from build123d import *

# Parameters (mm, degrees)
BOSS_EXTRUDE1_DEPTH      = 5
CUT_EXTRUDE1_DEPTH       = 1
BOSS_EXTRUDE2_DEPTH      = 0.0254
BOSS_EXTRUDE2_DEPTH_BACK = 1
SKETCH3_W                = 0.777152918
SKETCH3_H                = 1.679205413


with BuildPart() as part:
    # Sketch1 → Boss-Extrude1 (new body)
    with BuildSketch(Plane(origin=(0, 0, 0), x_dir=(1, 0, 0), z_dir=(0, 1, 0))):
        Polygon((-3, 2), (-2, 3), (2, 3), (3, 2), (3, -2), (2, -3), (-2, -3), (-3, -2), align=None)
    extrude(amount=BOSS_EXTRUDE1_DEPTH)

    # Sketch2 → Cut-Extrude1 (cut)
    with BuildSketch(Plane(origin=(0, 5, 0), x_dir=(1, 0, 0), z_dir=(0, 1, 0))):
        Polygon((3, -2), (3, 2), (2, 3), (-2, 3), (-3, 2), (-3, -2), (-2, -3), (2, -3), align=None)
        Polygon((2.492, -1.78957951), (2.492, 1.78957951), (1.78957951, 2.492), (-1.78957951, 2.492), (-2.492, 1.78957951), (-2.492, -1.78957951), (-1.78957951, -2.492), (1.78957951, -2.492), align=None, mode=Mode.SUBTRACT)
    extrude(amount=-CUT_EXTRUDE1_DEPTH, mode=Mode.SUBTRACT)

    # Sketch3 → Boss-Extrude2 (add, two sides: drawn at the far end of the back side and taken through both)
    with BuildSketch(Plane.XZ.offset(-BOSS_EXTRUDE2_DEPTH_BACK)):
        with Locations((0, 2.210397294)):
            Rectangle(SKETCH3_W, SKETCH3_H)
        with Locations((0, -2.210397294)):
            Rectangle(SKETCH3_W, SKETCH3_H)
    extrude(amount=BOSS_EXTRUDE2_DEPTH + BOSS_EXTRUDE2_DEPTH_BACK)


solid = part.part
The model under review builds one solid part; all positions refer to its coordinate system, in mm. A direction names the side the tool comes from. Give positions to 0.01 mm unless a question says otherwise; leave off trailing zeros. Order: outer loops, then holes, each group sorted by start corner. A loop starts at its lowest first (then second) coordinate and runs counter-clockwise, first axis right, second up. Notation, with made-up numbers: M 24,54.5 L 60,54.5 A33 cw 60,84.5 Z; hole C 61.5,-6.75 d10. An arc over 180 degrees is marked long. Answer in a Markdown table with one row per item. Add a question column.
1. Machinability: for faces 1 (the flat face through (2.492, 4.5, 0)), 2 (the flat face through (-2.492, 4.5, 0)), 3 (the flat face through (0, 4.5, 2.492)), 4 (the flat face through (0, 4.5, -2.492)), 5 (the flat face through (0, 4, -2.7)), which of the approach directions +Z, -Z, +X, -X, +Y, -Y give a long, thin tool a straight path to every point of the face, cutting with its end or side? Answer none if there is none.
2. Add section C-C on y = 4.45. State the section outline as (x, z) points, plus the area to 3 significant figures.
3. To check wall thickness, follow line 1 along Y through (x, z) = (-0.05, 1.25); line 2 along Z through (x, y) = (1.4, 1.3); line 3 along Z through (x, y) = (-0.15, 4.75). State the ranges of each line that lie inside material, in increasing order.
4. For pin 1 Ø3 at (x, z) = (2, -1.5) entering from -Y; pin 2 Ø0.5 at (y, z) = (4.5, 0) entering from +X; pin 3 Ø1.2 at (x, y) = (0.5, 3) entering from +Z, all flat-tipped, find the tip position at first contact; note any pin that passes through.
5. Add section D-D on x = 1.5. State the section outline as (y, z) points, plus the area to 3 significant figures.
The answers:
| question | item | result |
|---|---|---|
| 1 | face 1 | +Z, -Z, +X, +Y |
| 1 | face 2 | +Z, -Z, -X, +Y |
| 1 | face 3 | +Z, +X, -X, +Y |
| 1 | face 4 | -Z, +X, -X, +Y |
| 1 | face 5 | +Y |
| 2 | outline | M -2.49,-1.79 L -1.79,-2.49 L 1.79,-2.49 L 2.49,-1.79 L 2.49,1.79 L 1.79,2.49 L -1.79,2.49 L -2.49,1.79 Z |
| 2 | area | 23.9 mm2 |
| 3 | line 1 | 0 to 5 |
| 3 | line 2 | -3 to 3 |
| 3 | line 3 | -2.49 to 2.49 |
| 4 | pin 1 | y = 0 |
| 4 | pin 2 | x = 2.49 |
| 4 | pin 3 | z = 3 |
| 5 | outline | M 0,-3 L 4,-3 L 4,-2.49 L 5,-2.49 L 5,2.49 L 4,2.49 L 4,3 L 0,3 Z |
| 5 | area | 29.0 mm2 |
